from build123d import *

# Parameters (mm, degrees)
SPUR_START                = -38.37009116
SPUR_GEAR_ISO_OUTLINE_R   = 7
SPUR_GEAR_ISO_OUTLINE_R_2 = 5
SPUR_GEAR_ISO_DEPTH       = 24.0000508
SPUR_START_2              = -20.37004036
SPUR_GEAR_ISO_2_OUTLINE_R = 7
SPUR_GEAR_ISO_2_DEPTH     = 6
CUT_EXTRUDE1_DEPTH        = 5
BOSS_EXTRUDE1_START       = 2.5
SKETCH2_R                 = 7.749
SKETCH2_R_2               = 7
BOSS_EXTRUDE1_DEPTH       = 2.5


# Read off the part's stored shape, not the designer's step: spur gear_iso
with BuildPart() as part:
    # spur gear_iso outline → spur gear_iso (new body)
    with BuildSketch(Plane.YZ.offset(SPUR_START)):
        with Locations((4.178828844, 7.909958029)):
            Circle(SPUR_GEAR_ISO_OUTLINE_R)
        with Locations((4.178828844, 7.909958029)):
            Circle(SPUR_GEAR_ISO_OUTLINE_R_2, mode=Mode.SUBTRACT)
    extrude(amount=SPUR_GEAR_ISO_DEPTH)

    # spur gear_iso 2 outline → spur gear_iso 2 (add)
    with BuildSketch(Plane.YZ.offset(SPUR_START_2)):
        with BuildLine():
            ThreePointArc((10.863081906, 15.347750779), (10.606704941, 15.57040246), (10.342916446, 15.784221425))
            ThreePointArc((10.342916446, 15.784221425), (9.329220993, 15.189966754), (8.560887593, 14.300933081))
            ThreePointArc((8.560887593, 14.300933081), (8.053328844, 14.620788883), (7.522546219, 14.900419753))
            ThreePointArc((7.522546219, 14.900419753), (7.908305264, 16.010332833), (7.916097179, 17.185346182))
            ThreePointArc((7.916097179, 17.185346182), (7.599030277, 17.306884237), (7.278019782, 17.417587362))
            ThreePointArc((7.278019782, 17.417587362), (6.528704713, 16.512466369), (6.110774911, 15.414262487))
            ThreePointArc((6.110774911, 15.414262487), (5.524428573, 15.541233307), (4.930016667, 15.622462023))
            ThreePointArc((4.930016667, 15.622462023), (4.912898964, 16.797376517), (4.518342735, 17.904192883))
            ThreePointArc((4.518342735, 17.904192883), (4.178828843, 17.909958029), (3.839314952, 17.904192883))
            ThreePointArc((3.839314952, 17.904192883), (3.444758723, 16.797376517), (3.427641021, 15.622462023))
            ThreePointArc((3.427641021, 15.622462023), (2.833229115, 15.541233307), (2.246882776, 15.414262487))
            ThreePointArc((2.246882776, 15.414262487), (1.828952974, 16.512466369), (1.079637905, 17.417587362))
            ThreePointArc((1.079637905, 17.417587362), (0.75862741, 17.306884237), (0.441560508, 17.185346182))
            ThreePointArc((0.441560508, 17.185346182), (0.449352423, 16.010332833), (0.835111468, 14.900419753))
            ThreePointArc((0.835111468, 14.900419753), (0.304328844, 14.620788883), (-0.203229906, 14.300933081))
            ThreePointArc((-0.203229906, 14.300933081), (-0.971563306, 15.189966754), (-1.985258759, 15.784221425))
            ThreePointArc((-1.985258759, 15.784221425), (-2.249047253, 15.57040246), (-2.505424219, 15.347750779))
            ThreePointArc((-2.505424219, 15.347750779), (-2.09622398, 14.246264397), (-1.354116421, 13.335224631))
            ThreePointArc((-1.354116421, 13.335224631), (-1.757249546, 12.890919217), (-2.12480163, 12.416757764))
            ThreePointArc((-2.12480163, 12.416757764), (-3.150866281, 12.989390646), (-4.306675485, 13.201103111))
            ThreePointArc((-4.306675485, 13.201103111), (-4.481425194, 12.909958029), (-4.646189377, 12.613047801))
            ThreePointArc((-4.646189377, 12.613047801), (-3.884936401, 11.717943901), (-2.875989453, 11.115662288))
            ThreePointArc((-2.875989453, 11.115662288), (-3.102849275, 10.56027212), (-3.286062488, 9.988995885))
            ThreePointArc((-3.286062488, 9.988995885), (-4.446099849, 10.17616), (-5.604615157, 9.979794611))
            ThreePointArc((-5.604615157, 9.979794611), (-5.669248686, 9.646439806), (-5.722527095, 9.311082786))
            ThreePointArc((-5.722527095, 9.311082786), (-4.701039727, 8.730324108), (-3.546947281, 8.509444701))
            ThreePointArc((-3.546947281, 8.509444701), (-3.570171156, 7.909958029), (-3.546947281, 7.310471357))
            ThreePointArc((-3.546947281, 7.310471357), (-4.701039727, 7.089591951), (-5.722527095, 6.508833272))
            ThreePointArc((-5.722527095, 6.508833272), (-5.669248686, 6.173476252), (-5.604615157, 5.840121447))
            ThreePointArc((-5.604615157, 5.840121447), (-4.446099849, 5.643756058), (-3.286062488, 5.830920173))
            ThreePointArc((-3.286062488, 5.830920173), (-3.102849275, 5.259643938), (-2.875989453, 4.70425377))
            ThreePointArc((-2.875989453, 4.70425377), (-3.884936402, 4.101972158), (-4.646189377, 3.206868257))
            ThreePointArc((-4.646189377, 3.206868257), (-4.481425194, 2.909958029), (-4.306675485, 2.618812947))
            ThreePointArc((-4.306675485, 2.618812947), (-3.15086628, 2.830525412), (-2.12480163, 3.403158295))
            ThreePointArc((-2.12480163, 3.403158295), (-1.757249546, 2.928996842), (-1.354116421, 2.484691427))
            ThreePointArc((-1.354116421, 2.484691427), (-2.09622398, 1.573651661), (-2.505424219, 0.472165279))
            ThreePointArc((-2.505424219, 0.472165279), (-2.249047253, 0.249513598), (-1.985258759, 0.035694633))
            ThreePointArc((-1.985258759, 0.035694633), (-0.971563306, 0.629949304), (-0.203229906, 1.518982977))
            ThreePointArc((-0.203229906, 1.518982977), (0.304328844, 1.199127175), (0.835111468, 0.919496305))
            ThreePointArc((0.835111468, 0.919496305), (0.449352423, -0.190416775), (0.441560508, -1.365430124))
            ThreePointArc((0.441560508, -1.365430124), (0.75862741, -1.486968179), (1.079637905, -1.597671303))
            ThreePointArc((1.079637905, -1.597671303), (1.828952974, -0.69255031), (2.246882776, 0.405653572))
            ThreePointArc((2.246882776, 0.405653572), (2.833229115, 0.278682751), (3.427641021, 0.197454035))
            ThreePointArc((3.427641021, 0.197454035), (3.444758723, -0.977460459), (3.839314952, -2.084276825))
            ThreePointArc((3.839314952, -2.084276825), (4.178828843, -2.090041971), (4.518342735, -2.084276825))
            ThreePointArc((4.518342735, -2.084276825), (4.912898964, -0.977460459), (4.930016667, 0.197454035))
            ThreePointArc((4.930016667, 0.197454035), (5.524428573, 0.278682751), (6.110774911, 0.405653572))
            ThreePointArc((6.110774911, 0.405653572), (6.528704713, -0.69255031), (7.278019782, -1.597671303))
            ThreePointArc((7.278019782, -1.597671303), (7.599030277, -1.486968179), (7.916097179, -1.365430124))
            ThreePointArc((7.916097179, -1.365430124), (7.908305264, -0.190416775), (7.522546219, 0.919496305))
            ThreePointArc((7.522546219, 0.919496305), (8.053328844, 1.199127175), (8.560887593, 1.518982977))
            ThreePointArc((8.560887593, 1.518982977), (9.329220993, 0.629949304), (10.342916446, 0.035694633))
            ThreePointArc((10.342916446, 0.035694633), (10.606704941, 0.249513598), (10.863081906, 0.472165279))
            ThreePointArc((10.863081906, 0.472165279), (10.453881667, 1.573651661), (9.711774108, 2.484691427))
            ThreePointArc((9.711774108, 2.484691427), (10.114907233, 2.928996842), (10.482459318, 3.403158295))
            ThreePointArc((10.482459318, 3.403158295), (11.508523968, 2.830525412), (12.664333173, 2.618812947))
            ThreePointArc((12.664333173, 2.618812947), (12.839082882, 2.909958029), (13.003847064, 3.206868257))
            ThreePointArc((13.003847064, 3.206868257), (12.242594089, 4.101972158), (11.233647141, 4.70425377))
            ThreePointArc((11.233647141, 4.70425377), (11.460506962, 5.259643939), (11.643720175, 5.830920173))
            ThreePointArc((11.643720175, 5.830920173), (12.803757537, 5.643756058), (13.962272845, 5.840121447))
            ThreePointArc((13.962272845, 5.840121447), (14.026906374, 6.173476252), (14.080184782, 6.508833272))
            ThreePointArc((14.080184782, 6.508833272), (13.058697415, 7.089591951), (11.904604969, 7.310471357))
            ThreePointArc((11.904604969, 7.310471357), (11.927828844, 7.909958029), (11.904604969, 8.509444701))
            ThreePointArc((11.904604969, 8.509444701), (13.058697414, 8.730324108), (14.080184782, 9.311082786))
            ThreePointArc((14.080184782, 9.311082786), (14.026906374, 9.646439806), (13.962272845, 9.979794611))
            ThreePointArc((13.962272845, 9.979794611), (12.803757537, 10.17616), (11.643720175, 9.988995885))
            ThreePointArc((11.643720175, 9.988995885), (11.460506962, 10.56027212), (11.233647141, 11.115662288))
            ThreePointArc((11.233647141, 11.115662288), (12.242594089, 11.717943901), (13.003847064, 12.613047801))
            ThreePointArc((13.003847064, 12.613047801), (12.839082882, 12.909958029), (12.664333173, 13.201103111))
            ThreePointArc((12.664333173, 13.201103111), (11.508523969, 12.989390646), (10.482459318, 12.416757764))
            ThreePointArc((10.482459318, 12.416757764), (10.114907233, 12.890919217), (9.711774108, 13.335224631))
            ThreePointArc((9.711774108, 13.335224631), (10.453881667, 14.246264397), (10.863081906, 15.347750779))
        make_face()
        with Locations((4.178828844, 7.909958029)):
            Circle(SPUR_GEAR_ISO_2_OUTLINE_R, mode=Mode.SUBTRACT)
    extrude(amount=SPUR_GEAR_ISO_2_DEPTH)

    # Sketch1 → Cut-Extrude1 (cut)
    with BuildSketch(Plane.ZY.offset(38.37009116)):
        with BuildLine():
            ThreePointArc((1.072560864, 5.678828844), (0.909958029, 4.178828844), (1.072560864, 2.678828844))
            Line((1.072560864, 2.678828844), (1.909958029, 2.678828844))
            Line((1.909958029, 2.678828844), (1.909958029, 5.678828844))
            Line((1.909958029, 5.678828844), (1.072560864, 5.678828844))
        make_face()
        with BuildLine():
            Line((13.909958029, 2.678828844), (14.747355195, 2.678828844))
            ThreePointArc((14.747355195, 2.678828844), (14.869188596, 3.4244351), (14.909958029, 4.178828844))
            ThreePointArc((14.909958029, 4.178828844), (14.869188596, 4.933222587), (14.747355195, 5.678828844))
            Line((14.747355195, 5.678828844), (13.909958029, 5.678828844))
            Line((13.909958029, 5.678828844), (13.909958029, 2.678828844))
        make_face()
    extrude(amount=-CUT_EXTRUDE1_DEPTH, mode=Mode.SUBTRACT)

    # Sketch2 → Boss-Extrude1 (add)
    with BuildSketch(Plane.ZY.offset(20.37004036).offset(BOSS_EXTRUDE1_START)):
        with Locations((7.909958029, 4.178828844)):
            Circle(SKETCH2_R)
        with Locations(Location((7.909958029, 4.178828844, 0), (0, 0, 192.373625116))):
            Circle(SKETCH2_R_2, mode=Mode.SUBTRACT)
    extrude(amount=-BOSS_EXTRUDE1_DEPTH)


solid = part.part
Can you work these out from the model? Positions are in its coordinate system, mm. A direction names the side the tool comes from. Coordinates: 2 decimals unless noted, no trailing zeros. Order: outer loops, then holes, each group sorted by start corner. A loop starts at its lowest first (then second) coordinate and runs counter-clockwise, first axis right, second up. Notation, with made-up numbers: M 65,3.5 L 72,3.5 A17 ccw 72,36.5 Z; hole C 32,44 d4. An arc over 180 degrees is marked long. Answer as CSV lines item,"result".
(1) Suppose I cut it at B-B on x = -35.5. Please give me the cut outline in (y, z).
Geometry check:
outline,"M 2.68,1.07 L 2.68,1.91 L 5.68,1.91 L 5.68,1.07 A7 ccw 5.68,14.75 L 5.68,13.91 L 2.68,13.91 L 2.68,14.75 A7 ccw Z; hole C 4.18,7.91 d10"
(2) Please list where these lines run through material, in increasing order: L1, parallel to Y at x = -16, z = 14.75; L2, parallel to X at y = -3, z = 4.5; L3, parallel to X at y = 3.5, z = 0.25.
Geometry check:
L1,"-2.33 to -0.53, 0.54 to 7.82, 8.89 to 10.69"
L2,"-20.37 to -14.37"
L3,"-22.87 to -14.37"
(3) Suppose I cut it at C-C on z = 11.75. Please give me the cut outline in (x, y).
Geometry check:
outline,"M -38.37,-1.67 L -22.87,-1.67 L -22.87,-2.55 L -20.37,-2.55 L -20.37,-3.92 L -14.37,-3.92 L -14.37,0.98 L -38.37,0.98 Z; M -38.37,7.38 L -14.37,7.38 L -14.37,12.28 L -20.37,12.28 L -20.37,10.91 L -22.87,10.91 L -22.87,10.03 L -38.37,10.03 Z"
(4) On a 3-axis mill with a long thin cutter (end or side, diameter ignored), from which of +Z, -Z, +X, -X, +Y, -Y can I reach the whole of each face in a straight line? I mean faces 1 (the cylindrical face through (-17.412, 12.23, 11.707)), 2 (the flat face through (-20.37, -3.4, 3.4)), 3 (the flat face through (-20.37, -3, 12)), 4 (the cylindrical face through (-17.412, -4.717, 8.736)). Say none if no direction works.
Geometry check:
face 1,"+X, -X, +Y"
face 2,"-Z, -X, -Y"
face 3,"+Z, -X, -Y"
face 4,"+X, -X, -Y"
(5) I'm going to push flat-ended pins straight in: pin 1 (1.8 mm diameter, centred on y = -1, z = 15, fed in from -X); pin 2 (12 mm diameter, centred on x = -30.5, z = 1.5, fed in from -Y); pin 3 (3.5 mm diameter, centred on x = -36, y = 5, fed in from +Z); pin 4 (1 mm diameter, centred on y = 1.5, z = 10, fed in from +X). Where does each tip first touch, or does it pass through?
Geometry check:
pin 1,"x = -20.37"
pin 2,"y = -2.81"
pin 3,"z = 14.75"
pin 4,"through"
(6) Suppose I cut it at A-A on z = 7. Please give me the cut outline in (x, y).
Geometry check:
outline,"M -38.37,-2.76 L -22.87,-2.76 L -22.87,-3.52 L -20.37,-3.52 L -20.37,-4.92 L -14.37,-4.92 L -14.37,-0.74 L -38.37,-0.74 Z; M -38.37,9.1 L -14.37,9.1 L -14.37,13.28 L -20.37,13.28 L -20.37,11.87 L -22.87,11.87 L -22.87,11.12 L -38.37,11.12 Z"
(7) Suppose I cut it at D-D on x = -27.75. Please give me the cut outline in (y, z), plus the area to 3 significant figures.
Geometry check:
outline,"C 4.18,7.91 d14; hole C 4.18,7.91 d10"
area,"75.4 mm^2"
